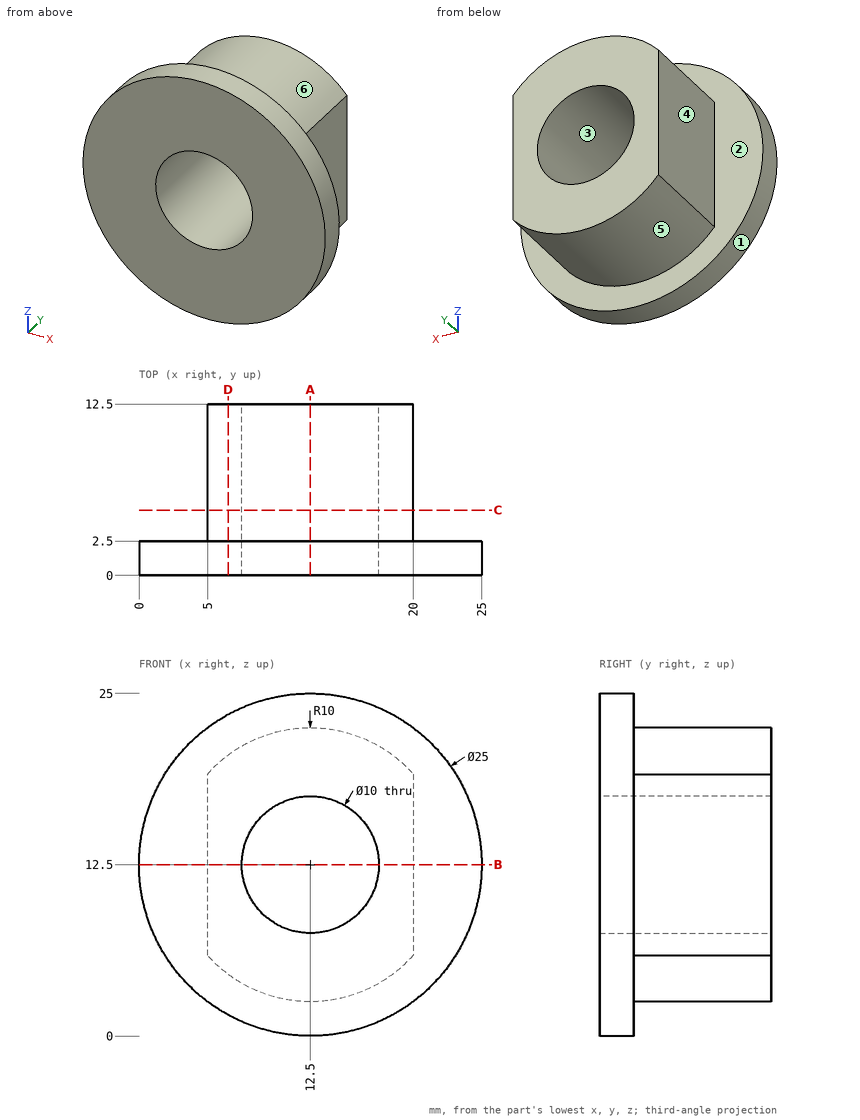
Job drawing, mm, ordinate dimensions from the low corner. One solid piece. A direction names the side the tool comes from. Round coordinates to 2 decimals unless told otherwise and drop trailing zeros. Order: outer loops, then holes, each group sorted by start corner. A loop starts at its lowest first (then second) coordinate and runs counter-clockwise, first axis right, second up. Notation, with made-up numbers: (-36.5, -5) -> (6.5, -5) arc R16 ccw to (6.5, 10) -> close; hole circle Ø4 at (62, 76.5). An arc over 180 degrees is marked (long way). Answer in a Markdown table with one row per item.
1) Band-saw the part on C-C on y = 4.75. Give the cut face in (x, z), and give its area (3 significant figures).
Values:
| item | result |
|---|---|
| outline | (5, 5.89) arc R10 ccw to (20, 5.89) -> (20, 19.11) arc R10 ccw to (5, 19.11) -> close; hole circle Ø10 at (12.5, 12.5) |
| area | 190 mm2 |
2) Pin check, flat tips, straight feed: P1, Ø1.5, axis at x = 13.5, y = 1.5, coming from the +Z side; P2, Ø1.5, axis at x = 16.5, y = 5.5, coming from the +Z side; P3, Ø9, axis at x = 12.5, z = 12.5, coming from the -Y side; P4, Ø2, axis at y = 9.5, z = 21, coming from the -X side. Stop position of each tip, or through.
Values:
| item | result |
|---|---|
| P1 | z = 25 |
| P2 | z = 21.96 |
| P3 | through |
| P4 | x = 5.89 |
3) Band-saw the part on A-A on x = 12.5. Give the cut face in (y, z).
Values:
| item | result |
|---|---|
| outline | (0, 0) -> (2.5, 0) -> (2.5, 2.5) -> (12.5, 2.5) -> (12.5, 7.5) -> (0, 7.5) -> close; (0, 17.5) -> (12.5, 17.5) -> (12.5, 22.5) -> (2.5, 22.5) -> (2.5, 25) -> (0, 25) -> close |
4) Which spindle directions (+Z, -Z, +X, -X, +Y, -Y) get a long thin tool onto all of the face, cutting with end or side? Do the marked faces 4, 5 and 6. Say none if no direction does.
Values:
| item | result |
|---|---|
| face 4 | +Z, -Z, -X, +Y |
| face 5 | -Z, +Y |
| face 6 | +Z, +Y |
5) Band-saw the part on B-B on z = 12.5. Give the cut face in (x, y).
Values:
| item | result |
|---|---|
| outline | (0, 0) -> (7.5, 0) -> (7.5, 12.5) -> (5, 12.5) -> (5, 2.5) -> (0, 2.5) -> close; (17.5, 0) -> (25, 0) -> (25, 2.5) -> (20, 2.5) -> (20, 12.5) -> (17.5, 12.5) -> close |
6) Wall check: L1, parallel to X at y = 7.25, z = 12.5; L2, parallel to Z at x = 12.75, y = 6.5; L3, parallel to Y at x = 16.75, z = 1. Give the ranges that are in metal, low to high.
Values:
| item | result |
|---|---|
| L1 | 5 to 7.5, 17.5 to 20 |
| L2 | 2.5 to 7.51, 17.49 to 22.5 |
| L3 | 0 to 2.5 |
7) Band-saw the part on D-D on x = 6.5. Give the cut face in (y, z).
Values:
| item | result |
|---|---|
| outline | (0, 1.53) -> (2.5, 1.53) -> (2.5, 4.5) -> (12.5, 4.5) -> (12.5, 20.5) -> (2.5, 20.5) -> (2.5, 23.47) -> (0, 23.47) -> close |
8) Mould opens along X. For the marked faces 1, 2 and 3 say: released by +X, released by -X, zero draft, split by the parting line, or undercut.
Values:
| item | result |
|---|---|
| face 1 | split by the parting line |
| face 2 | zero draft |
| face 3 | undercut |
